```python
from build123d import *

# Parameters (mm, degrees)
BOSS_EXTRUDE1_DEPTH            = 130.5
SKETCH4_W                      = 34.8
SKETCH4_H                      = 34.8
SKETCH4_R                      = 13.45
BOSS_EXTRUDE2_DEPTH            = 130.5
FILLET1_R                      = 5
CUT_EXTRUDE4_DEPTH             = 182.887575167
CUT_EXTRUDE5_REACH             = 226.442
SKETCH7_R                      = 8.2
CUT_EXTRUDE5_DIRECTION_2_REACH = 226.442
SKETCH8_R                      = 13.55
CUT_EXTRUDE6_DEPTH             = 182.887575238


with BuildPart() as part:
    # Sketch1 → Boss-Extrude1 (new body)
    with BuildSketch(Plane(origin=(0, 0, 0), x_dir=(1, 0, 0), z_dir=(0, 1, 0))):
        with BuildLine():
            Line((0, 0), (-34, 0))
            Line((-34, 0), (-100, -43))
            Line((-100, -43), (-100, -66.97))
            Line((-100, -66.97), (-97.358644924, -66.97))
            ThreePointArc((-97.358644924, -66.97), (-95.748804634, -66.156766295), (-95.448140727, -64.378414239))
            ThreePointArc((-95.448140727, -64.378414239), (-82.6, -46.95), (-69.751859273, -64.378414239))
            ThreePointArc((-69.751859273, -64.378414239), (-69.451195366, -66.156766295), (-67.841355076, -66.97))
            Line((-67.841355076, -66.97), (-65.2, -66.97))
            Line((-65.2, -66.97), (-65.2, -43))
            Line((-65.2, -43), (-34, -3))
            Line((-34, -3), (0, -3))
            Line((0, -3), (0, 0))
        make_face()
        Polygon((-69.004681327, -43), (-94.504291462, -43), (-42.656655328, -9.220479488), align=None, mode=Mode.SUBTRACT)
    boss_extrude1 = extrude(amount=BOSS_EXTRUDE1_DEPTH)

    # Mirror1: Boss-Extrude1 across plane
    add(boss_extrude1.mirror(Plane(origin=(0, 130.5, 3), x_dir=(0, 0, 1), z_dir=(-1, 0, 0))))

    # Sketch4 → Boss-Extrude2 (add)
    with BuildSketch(Plane.XZ):
        with Locations((82.6, 60.4)):
            Rectangle(SKETCH4_W, SKETCH4_H)
        with Locations(Location((82.6, 60.4, 0), (0, 0, 270))):
            Circle(SKETCH4_R, mode=Mode.SUBTRACT)
    extrude(amount=-BOSS_EXTRUDE2_DEPTH)

    # Fillet1
    fillet1_edges = [part.edges().sort_by_distance(p)[0] for p in [
        (-34, 65.25, 3),
        (-65.2, 65.25, 43),
        (-100, 65.25, 43),
        (-34, 65.25, 0),
        (34, 65.25, 3),
        (65.2, 65.25, 43),
        (100, 65.25, 43),
        (34, 65.25, 0),
    ]]
    fillet(fillet1_edges, radius=FILLET1_R)

    # Sketch5 → Cut-Extrude4 (cut, through all)
    with BuildSketch(Plane.XZ):
        with BuildLine():
            Line((65.2, 60.4), (65.2, 77.8))
            Line((65.2, 77.8), (83.070170915, 82.404410021))
            Line((83.070170915, 82.404410021), (100, 77.8))
            Line((100, 77.8), (100, 60.4))
            ThreePointArc((100, 60.4), (82.6, 77.8), (65.2, 60.4))
        make_face()
    extrude(amount=-CUT_EXTRUDE4_DEPTH, mode=Mode.SUBTRACT)

    # Sketch7 → Cut-Extrude5 (cut, up to next)
    with BuildSketch(Plane.ZY.offset(-65.2), mode=Mode.PRIVATE) as cut_extrude5_sk1:
        with Locations((34.8, 0)):
            Circle(SKETCH7_R)
    cut_extrude5_tool1 = extrude(cut_extrude5_sk1.sketch, amount=-CUT_EXTRUDE5_REACH, mode=Mode.PRIVATE) & part.part
    # Sketch7 → Cut-Extrude5 (cut, up to next)
    with BuildSketch(Plane.ZY.offset(-65.2), mode=Mode.PRIVATE) as cut_extrude5_sk2:
        with Locations((34.8, 130.5)):
            Circle(SKETCH7_R)
    cut_extrude5_tool2 = extrude(cut_extrude5_sk2.sketch, amount=-CUT_EXTRUDE5_REACH, mode=Mode.PRIVATE) & part.part
    add(cut_extrude5_tool1.solids().sort_by_distance((65.2, 0, 34.8))[0], mode=Mode.SUBTRACT)
    add(cut_extrude5_tool2.solids().sort_by_distance((65.2, 130.5, 34.8))[0], mode=Mode.SUBTRACT)

    # Sketch7 → Cut-Extrude5 direction 2 (cut, up to next)
    with BuildSketch(Plane.ZY.offset(-65.2), mode=Mode.PRIVATE) as cut_extrude5_direction_2_sk1:
        with Locations((34.8, 0)):
            Circle(SKETCH7_R)
    cut_extrude5_direction_2_tool1 = extrude(cut_extrude5_direction_2_sk1.sketch, amount=CUT_EXTRUDE5_DIRECTION_2_REACH, mode=Mode.PRIVATE) & part.part
    # Sketch7 → Cut-Extrude5 direction 2 (cut, up to next)
    with BuildSketch(Plane.ZY.offset(-65.2), mode=Mode.PRIVATE) as cut_extrude5_direction_2_sk2:
        with Locations((34.8, 130.5)):
            Circle(SKETCH7_R)
    cut_extrude5_direction_2_tool2 = extrude(cut_extrude5_direction_2_sk2.sketch, amount=CUT_EXTRUDE5_DIRECTION_2_REACH, mode=Mode.PRIVATE) & part.part
    add(cut_extrude5_direction_2_tool1.solids().sort_by_distance((65.2, 0, 34.8))[0], mode=Mode.SUBTRACT)
    add(cut_extrude5_direction_2_tool2.solids().sort_by_distance((65.2, 130.5, 34.8))[0], mode=Mode.SUBTRACT)

    # Sketch8 → Cut-Extrude6 (cut, through all)
    with BuildSketch(Plane.XZ):
        with Locations(Location((82.6, 60.4, 0), (0, 0, 270))):
            Circle(SKETCH8_R)
    extrude(amount=-CUT_EXTRUDE6_DEPTH, mode=Mode.SUBTRACT)


solid = part.part
```
For this review, take the finished solid that the model builds, in its own axes (mm). A direction names the side the tool comes from. Round coordinates to 2 decimals unless told otherwise and drop trailing zeros. Order: outer loops, then holes, each group sorted by start corner. A loop starts at its lowest first (then second) coordinate and runs counter-clockwise, first axis right, second up.
Q1. Mouldability with a two-part tool opening along X and no side actions: class faces 4 (the cylindrical face through (91.758, 64.336, 70.387)), 5 (the flat face through (100, 64, 53)), 6 (the cylindrical face through (-99.38, 66.16, 43.3)), 7 (the cylindrical face through (33.72, 66.16, 3.49)) as pulls with the +X half, pulls with the -X half, needs draft (parallel to the pull), parting line crosses it, or undercut.
Findings below:
face 4: undercut
face 5: pulls with the +X half
face 6: pulls with the -X half
face 7: undercut
Q2. We need section C-C, the plane z = 36. Give the boundary of the cut face in (x, y).
Findings below:
outline: (-89.26, 0) - (-83.76, 0) - (-83.76, 130.5) - (-89.26, 130.5) - close; (-63.54, 0) - (-59.74, 0) - (-59.74, 130.5) - (-63.54, 130.5) - close; (59.74, 8.11) - (63.54, 8.11) - (63.54, 122.39) - (59.74, 122.39) - close; (83.76, 0) - (89.26, 0) - (89.26, 130.5) - (83.76, 130.5) - close
Q3. Machinability: for faces 1 (the flat face through (-100, 64, 56)), 2 (the flat face through (-50.02, 64.34, 23.54)), 3 (the flat face through (68.943, 64.336, 26.347)), which of the approach directions +Z, -Z, +X, -X, +Y, -Y give a long, thin tool a straight path to every point of the face, cutting with its end or side? Answer none if there is none.
Findings below:
face 1: +Z, -Z, -X, +Y, -Y
face 2: +Z, +Y, -Y
face 3: +Y, -Y
Q4. We need section B-B, the plane y = 63.5. State how many separate pieces and enclosed holes the cut face has, plus the area to 3 significant figures.
Findings below:
separate pieces: 1
enclosed holes: 3
area: 1,810 mm2
Q5. We need section A-A, the plane x = -82.6. Give the boundary of the cut face in (y, z), plus the area to 3 significant figures.
Findings below:
outline: (0, 31.66) - (130.5, 31.66) - (130.5, 35.24) - (0, 35.24) - close; (0, 43) - (130.5, 43) - (130.5, 46.95) - (0, 46.95) - close
area: 983 mm2
Q6. We need section D-D, the plane z = 7. Give the boundary of the cut face in (x, y), plus the area to 3 significant figures.
Findings below:
outline: (-44.74, 0) - (-37.12, 0) - (-37.12, 130.5) - (-44.74, 130.5) - close; (37.12, 0) - (44.74, 0) - (44.74, 130.5) - (37.12, 130.5) - close
area: 1,990 mm2
Q7. Insertion check: P1, Ø2, axis at y = 112, z = 16.5, coming from the +X side; P2, Ø4, axis at x = 48, y = 112, coming from the +Z side; P3, Ø7.5, axis at x = 77, y = 37, coming from the -Z side. Each pin has a flat end and moves straight along its axis. Give the tip position at first contact, or say it passes through.
Findings below:
P1: stops at x = 60.86
P2: stops at z = 23.51
P3: stops at z = 25.57
Q8. Wall thickness on line 1 (X direction, y = 52, z = 60); line 2 (X direction, y = 115.5, z = 9.5); line 3 (Z direction, x = -82.6, y = 45): over which ranges is each line inside the solid? List them lowest first.
Findings below:
line 1: x = -100 to -96.04, -69.16 to -65.2, 65.2 to 69.06, 96.14 to 100
line 2: x = -48.58 to -43.09, -42.87 to -39.07, 39.07 to 42.87, 43.09 to 48.58
line 3: z = 31.66 to 35.24, 43 to 46.95
